Source: CAD feature listing. Evaluate the final solid. Frame: model axes, mm. Give positions to 0.01 mm unless a question says otherwise; leave off trailing zeros. Write each loop counter-clockwise with the first axis right and the second up, starting at its lowest first coordinate (ties: lowest second). Pieces come first, ordered by that corner, then holes. Notation, with made-up numbers: (39, 77) -> (45, 77) arc R9 cw to (45, 94) -> close; hole circle Ø10 at (17, 85.25). An arc over 180 degrees is marked (long way). Answer as a JSON object with one key per item and string values. Group by question number.
Item 1: Pull-direction query (X, two-part tool) for faces 1 (the face through (-68, 100, 0)), 2 (the face through (-3.07, 2.82, 3.13)), 3 (the face through (-278.84, 173.39, 3.13)); classes: pulls with the +X half, pulls with the -X half, needs draft (parallel to the pull), parting line crosses it, or undercut.
Item 2: Section query D-D on x = 120.5. Return the cut outline in (y, z).
Item 3: First-contact query: pin 1 Ø3 at (x, z) = (-206, 4.5) entering from -Y; pin 2 Ø1 at (y, z) = (92.5, 4.5) entering from -X. Flat tips, straight axial feed; report the tip coordinate or a pass-through.
Item 4: Section query C-C on y = 0. Return the cut outline in (x, z), plus the area to 3 significant figures.
Item 5: Ray query, probe 1 along X at (y, z) = (-1, 1); probe 2 along Y at (x, z) = (111.5, 1.5); probe 3 along Y at (x, z) = (-134.5, 2). Return the intervals inside material, ascending. Write a range as from..to.
Item 6: Section query A-A on x = 35. Return the cut outline in (y, z) (3 decimals), plus the area to 3 significant figures.
Item 7: Section query B-B on z = 2.5. Return the cut outline in (x, y) (3 decimals).
from build123d import *

# Parameters (mm, degrees)
CROQUIS1_W              = 62
CROQUIS1_H              = 44.45
CROQUIS1_R              = 4.168993309
SALIENTE_EXTRUIR1_DEPTH = 6.35
CORTAR_EXTRUIR1_DEPTH   = 6.35
CROQUIS4_W              = 501.85323645
CROQUIS4_H              = 287.183942178
CORTAR_EXTRUIR2_DEPTH   = 6.35


with BuildPart() as part:
    # Croquis1 → Saliente-Extruir1 (new body)
    # profile 1 of 2: a face of its own
    with BuildSketch(Plane.XY):
        with BuildLine():
            Line((31, 22.225), (31, -22.225))
            Line((31, -22.225), (333, -22.225))
            ThreePointArc((333, -22.225), (468.296416477, 31.525514455), (581.256141711, 123.364169664))
            ThreePointArc((581.256141711, 123.364169664), (583.174687818, 126.479763895), (583.844075147, 130.076938784))
            Line((583.844075147, 130.076938784), (583.844075147, 166.244969995))
            ThreePointArc((583.844075147, 166.244969995), (580.915142959, 173.316037807), (573.844075147, 176.244969995))
            Line((573.844075147, 176.244969995), (-271.844075147, 176.244969995))
            ThreePointArc((-271.844075147, 176.244969995), (-278.915142959, 173.316037807), (-281.844075147, 166.244969995))
            Line((-281.844075147, 166.244969995), (-281.844075147, 130.076938784))
            ThreePointArc((-281.844075147, 130.076938784), (-281.174687818, 126.479763895), (-279.256141711, 123.364169664))
            ThreePointArc((-279.256141711, 123.364169664), (-166.296416477, 31.525514455), (-31, -22.225))
            Line((-31, -22.225), (-31, 22.225))
            Line((-31, 22.225), (31, 22.225))
        make_face()
    # profile 2 of 2: a face of its own
    with BuildSketch(Plane.XY):
        Rectangle(CROQUIS1_W, CROQUIS1_H)
        Circle(CROQUIS1_R, mode=Mode.SUBTRACT)
    extrude(amount=SALIENTE_EXTRUIR1_DEPTH)

    # Croquis3 → Cortar-Extruir1 (cut)
    with BuildSketch(Plane.XY.offset(6.35)):
        with BuildLine():
            Line((151, -22.225), (151, 70))
            Line((151, 70), (0, 70))
            ThreePointArc((0, 70), (56.814390783, 40.891625059), (66.378079025, -22.225))
            Line((66.378079025, -22.225), (151, -22.225))
        make_face()
        with BuildLine():
            Line((302, 70), (151, 70))
            Line((151, 70), (151, -22.225))
            Line((151, -22.225), (235.621920975, -22.225))
            ThreePointArc((235.621920975, -22.225), (245.185609217, 40.891625059), (302, 70))
        make_face()
    extrude(amount=-CORTAR_EXTRUIR1_DEPTH, mode=Mode.SUBTRACT)

    # Croquis4 → Cortar-Extruir2 (cut)
    with BuildSketch(Plane.XY.offset(6.35)):
        with Locations((401.926618225, 32.652998906)):
            Rectangle(CROQUIS4_W, CROQUIS4_H)
    extrude(amount=-CORTAR_EXTRUIR2_DEPTH, mode=Mode.SUBTRACT)


solid = part.part
Worked answers:
{
 "1": {"face 1": "needs draft", "face 2": "undercut", "face 3": "pulls with the -X half"},
 "2": {"outline": "(70, 0) -> (176.24, 0) -> (176.24, 6.35) -> (70, 6.35) -> close"},
 "3": {"pin 1": "y = 56.44", "pin 2": "x = -249.19"},
 "4": {"outline": "(-101.97, 0) -> (-4.17, 0) -> (-4.17, 6.35) -> (-101.97, 6.35) -> close; (4.17, 0) -> (70, 0) -> (70, 6.35) -> (4.17, 6.35) -> close", "area": "1,040 mm^2"},
 "5": {"probe 1": "-99.46..-4.05, 4.05..69.99", "probe 2": "70..176.24", "probe 3": "14.45..176.24"},
 "6": {"outline": "(-22.225, 0) -> (60.622, 0) -> (60.622, 6.35) -> (-22.225, 6.35) -> close; (70, 0) -> (176.245, 0) -> (176.245, 6.35) -> (70, 6.35) -> close", "area": "1,200 mm^2"},
 "7": {"outline": "(-281.844, 130.077) arc R10 ccw to (-279.256, 123.364) arc R480 ccw to (-31, -22.225) -> (66.378, -22.225) arc R70 ccw to (0, 70) -> (151, 70) -> (151, 176.245) -> (-271.844, 176.245) arc R10 ccw to (-281.844, 166.245) -> close; hole circle Ø8.338 at (0, 0)"}
}
